Geometry check sheet. Reference: the model listing, model coordinates, mm. A direction names the side the tool comes from. Give positions to 0.01 mm unless a question says otherwise; leave off trailing zeros. Write each loop counter-clockwise with the first axis right and the second up, starting at its lowest first coordinate (ties: lowest second). Pieces come first, ordered by that corner, then holes.
(1) Tool access check on faces 4 (the flat face through (-10.835, 60, -38)), 5 (the flat face through (29, 25, -61.5)), 6 (the flat face through (-20, 60, -13.5)), 7 (the flat face through (30, 40, 62)), 8 (the flat face through (31, 20, -78)). Record the directions out of +Z, -Z, +X, -X, +Y, -Y that give a thin tool (end or side, any length) a straight path to the whole face; none if there is none.
(2) Cross-section at D-D (z = -91.5). Record the boundary of the cut face in (x, y) (3 decimals).
(3) Thickness scan on line 1 along Z through (x, y) = (39.5, 38.5); line 2 along X through (y, z) = (53.5, -35.5) (3 decimals); line 3 along X through (y, z) = (32, -51.5) (3 decimals). Record the ranges inside material, lowest first.
(4) Cross-section at A-A (y = 71.5). Record the boundary of the cut face in (x, z) (3 decimals), and give its area (3 significant figures).
(5) Cross-section at B-B (z = -31). Record the boundary of the cut face in (x, y) (3 decimals), and give its area (3 significant figures).
(6) Mould release check, pull along X, two halves, no side actions. Record for faces 1 (the flat face through (70, 45, 50)), 2 (the flat face through (31, 20, 87)), 3 (the flat face through (-29.875, 60, -37)): +X half, -X half, draft (parallel to the pull), parting line (faces both ways), or undercut.
(7) Cross-section at C-C (y = 30). Record the boundary of the cut face in (x, z) (3 decimals), and give its area (3 significant figures).
(8) Depth check by flat-ended pin: P1, Ø4, axis at x = 91.5, y = 30, coming from the +Z side; P2, Ø10, axis at y = 61, z = 48.5, coming from the +X side (3 decimals); P3, Ø7, axis at y = 49.5, z = 61.5, coming from the -X side (3 decimals). Enter the tip coordinate at first touch or a pass-through.
Autodesk Inventor part; units mm, degrees
ref_plane "YZ Plane" through (0, 0, 0) normal (1, 0, 0) x (0, 1, 0)
ref_plane "XZ Plane" through (0, 0, 0) normal (0, 1, 0) x (-1, 0, 0)
ref_plane "XY Plane" through (0, 0, 0) normal (0, 0, 1) x (1, 0, 0)
sketch "Sketch1" plane through (0, 0, 0) normal (0, 1, 0) x (-1, 0, 0)
  line L0 (49.875, 66.5) -> (-110.125, 66.5)
  line L1 (-110.125, 66.5) -> (-110.125, -66.5)
  line L2 (-110.125, -66.5) -> (49.875, -66.5)
  line L3 (49.875, -66.5) -> (49.875, 66.5)
  line L4 (24.875, -66.5) -> (-85.125, -66.5)
  line L5 (-85.125, -66.5) -> (-85.125, -219)
  line L6 (-85.125, -219) -> (24.875, -219)
  line L7 (24.875, -219) -> (24.875, -66.5)
  point P0 (0, 0)
  dimension "d0" = 133
  dimension "d1" = 160
  dimension "d2" = 25
  dimension "d3" = 25
  dimension "d4" = 110
extrude "Extrusion1" add sketch "Sketch1" along normal blind 40 contours L3 L2 L1 L0
sketch "Sketch2" plane through (0, 40, 0) normal (0, 1, 0) x (1, 0, 0)
  line L0 (110.125, 66.5) -> (-49.875, 66.5) construction
  line L1 (-49.875, 66.5) -> (-49.875, -66.5) construction
  line L2 (-49.875, -66.5) -> (110.125, -66.5) construction
  line L3 (110.125, -66.5) -> (110.125, 66.5) construction
  line L4 (-29.875, 66.5) -> (-10.8349, 66.5)
  line L5 (-10.8349, 66.5) -> (-10.8349, 13.5)
  line L6 (-10.8349, 13.5) -> (-29.875, 13.5)
  line L7 (-29.875, 13.5) -> (-29.875, 66.5)
  line L8 (90.125, 66.5) -> (69.2723, 66.5)
  line L9 (69.2723, 66.5) -> (69.2723, 13.5)
  line L10 (69.2723, 13.5) -> (90.125, 13.5)
  line L11 (90.125, 13.5) -> (90.125, 66.5)
  line L12 (-32.3584, 66.5) -> (100, 66.5)
  line L13 (100, 66.5) -> (100, 61.5)
  line L14 (100, 61.5) -> (-32.3584, 61.5)
  line L15 (-32.3584, 61.5) -> (-32.3584, 66.5)
  point P0 (0, 0)
  point P1 (-10.8349, 61.5)
  point P2 (-29.875, 61.5)
  point P3 (90.125, 61.5)
  point P4 (69.2723, 61.5)
  point P5 (-27, 66.5)
  dimension "d7" = 20
  dimension "d8" = 20
  dimension "d11" = 80
  dimension "d12" = 80
  dimension "d13" = 120
  dimension "d35" = 5
extrude "Extrusion2" add sketch "Sketch2" along normal blind 40 contours L14 L5 L6 L7 | L14 L11 L10 L9
sketch "Sketch3" plane through (0, 40, 0) normal (0, 1, 0) x (1, 0, 0)
  line L0 (90.125, 61.5) -> (90.125, 13.5) construction
  line L1 (90.125, 13.5) -> (69.2723, 13.5) construction
  line L2 (69.2723, 13.5) -> (69.2723, 61.5) construction
  line L3 (-10.8349, 61.5) -> (-10.8349, 13.5) construction
  line L4 (-10.8349, 13.5) -> (-29.875, 13.5) construction
  line L5 (-29.875, 13.5) -> (-29.875, 61.5) construction
  line L6 (-49.875, 66.5) -> (-49.875, -66.5) construction
  line L7 (-49.875, -66.5) -> (110.125, -66.5) construction
  line L8 (110.125, -66.5) -> (110.125, 66.5) construction
  line L9 (-39.875, -56.5) -> (-39.875, 56.5)
  line L10 (-39.875, 56.5) -> (-34.875, 56.5)
  line L11 (-34.875, 56.5) -> (-34.875, 8.5)
  line L12 (-34.875, 8.5) -> (-5.8349, 8.5)
  line L13 (-5.8349, 8.5) -> (-5.8349, 61.5)
  line L14 (-5.8349, 61.5) -> (64.2723, 61.5)
  line L15 (64.2723, 61.5) -> (64.2723, 8.5)
  line L16 (64.2723, 8.5) -> (95.125, 8.5)
  line L17 (95.125, 8.5) -> (95.125, 56.5)
  line L18 (95.125, 56.5) -> (100.125, 56.5)
  line L19 (100.125, 56.5) -> (100.125, -56.5)
  line L20 (100.125, -56.5) -> (-39.875, -56.5)
  line L21 (-29.875, 61.5) -> (-10.8349, 61.5)
  line L22 (69.2723, 61.5) -> (90.125, 61.5)
  line L23 (110.125, 66.5) -> (-49.875, 66.5)
  point P0 (0, 0)
  dimension "d16" = 10
extrude "Extrusion3" cut sketch "Sketch3" against normal blind 30
sketch "Sketch4" plane through (0, 40, 0) normal (0, 1, 0) x (1, 0, 0)
  line L0 (-49.875, 66.5) -> (-49.875, -66.5) construction
  line L1 (-49.875, -66.5) -> (110.125, -66.5) construction
  line L2 (110.125, -66.5) -> (110.125, 66.5) construction
  line L3 (-35.875, -66.5) -> (16.125, -66.5)
  line L4 (16.125, -66.5) -> (16.125, -52)
  line L5 (16.125, -52) -> (-35.875, -52)
  line L6 (-35.875, -52) -> (-35.875, -66.5)
  line L7 (96.125, -66.5) -> (44.125, -66.5)
  line L8 (44.125, -66.5) -> (44.125, -50)
  line L9 (44.125, -50) -> (96.125, -50)
  line L10 (96.125, -50) -> (96.125, -66.5)
  point P0 (0, 0)
  dimension "d19" = 28
  dimension "d20" = 14
  dimension "d21" = 14
  dimension "d24" = 52
  dimension "d25" = 52
extrude "Extrusion4" add sketch "Sketch4" along normal mid plane 80
sketch "Sketch5" plane through (110.125, 0, 66.5) normal (1, 0, 0) x (0, 0, -1)
  line L0 (133, 0) -> (133, 40) construction
  line L1 (133, 0) -> (173, 0)
  line L2 (173, 0) -> (173, 20)
  line L3 (173, 20) -> (133, 20)
  line L4 (133, 20) -> (133, 0)
  line L5 (0, 0) -> (-40, 0)
  line L6 (-40, 0) -> (-40, 20)
  line L7 (-40, 20) -> (0, 20)
  line L8 (0, 20) -> (0, 0)
  point P0 (66.5, 0)
  dimension "d26" = 20
  dimension "d27" = 40
  dimension "d30" = 40
extrude "Extrusion5" add sketch "Sketch5" against normal up to surface (160 mm away)
sketch "Sketch6" plane through (0, 0, 0) normal (0, -1, 0) x (1, 0, 0)
  line L0 (110.125, -106.5) -> (-49.875, -106.5) construction
  circle A0 centre (30.125, -206.5) radius 125
  point P0 (0, 0)
  dimension "d31" = 100
  dimension "d32" = 250
extrude "Extrusion6" cut sketch "Sketch6" against normal blind 100
sketch "Sketch7" plane through (0, 80, 0) normal (0, 1, 0) x (1, 0, 0)
  point P0 (0, 0)
properties part number "FlanecForwardBabka"
Reply:
1. face 4: -Z, +Y
1. face 5: +Y
1. face 6: +X, -X, +Y
1. face 7: +Z, -Z, +Y
1. face 8: -Z, +X, -X, +Y
2. outline: (-49.875, 0) - (-18.865, 0) - (-18.865, 20) - (-49.875, 20) - close; (79.115, 0) - (110.125, 0) - (110.125, 20) - (79.115, 20) - close
3. line 1: z = -66.5 to -61.5, 56.5 to 66.5
3. line 2: x = -29.875 to -10.835, 69.272 to 90.125
3. line 3: x = -49.875 to -39.875, -34.875 to -5.835, 64.272 to 95.125, 100.125 to 110.125
4. outline: (-35.875, 52) - (16.125, 52) - (16.125, 66.5) - (-35.875, 66.5) - close; (-29.875, -61.5) - (-10.835, -61.5) - (-10.835, -13.5) - (-29.875, -13.5) - close; (44.125, 50) - (96.125, 50) - (96.125, 66.5) - (44.125, 66.5) - close; (69.272, -61.5) - (90.125, -61.5) - (90.125, -13.5) - (69.272, -13.5) - close
4. area: 3,530 mm2
5. outline: (-49.875, 0) - (110.125, 0) - (110.125, 40) - (100.125, 40) - (100.125, 10) - (95.125, 10) - (95.125, 40) - (90.125, 40) - (90.125, 80) - (69.272, 80) - (69.272, 40) - (64.272, 40) - (64.272, 10) - (-5.835, 10) - (-5.835, 40) - (-10.835, 40) - (-10.835, 80) - (-29.875, 80) - (-29.875, 40) - (-34.875, 40) - (-34.875, 10) - (-39.875, 10) - (-39.875, 40) - (-49.875, 40) - close
5. area: 5,590 mm2
6. face 1: undercut
6. face 2: draft
6. face 3: -X half
7. outline: (-49.875, -66.5) - (110.125, -66.5) - (110.125, 66.5) - (-49.875, 66.5) - close; hole (-39.875, -56.5) - (-34.875, -56.5) - (-34.875, -8.5) - (-5.835, -8.5) - (-5.835, -61.5) - (64.272, -61.5) - (64.272, -8.5) - (95.125, -8.5) - (95.125, -56.5) - (100.125, -56.5) - (100.125, 56.5) - (96.125, 56.5) - (96.125, 50) - (44.125, 50) - (44.125, 56.5) - (16.125, 56.5) - (16.125, 52) - (-35.875, 52) - (-35.875, 56.5) - (-39.875, 56.5) - close
7. area: 8,560 mm2
8. P1: stops at z = 66.5
8. P2: stops at x = 96.125
8. P3: stops at x = -35.875
